```python
from build123d import *

# Parameters (mm, degrees)
F0_W     = 115
F0_H     = 65
F1_DEPTH = 5
F2_DEPTH = 5
F3_DEPTH = 10


with BuildPart() as f1:
    # F0 (on Top) → F1 (new body)
    with BuildSketch(Plane.XY):
        with Locations((-62.5, 32.5)):
            Rectangle(F0_W, F0_H)
    extrude(amount=F1_DEPTH)



with BuildPart() as f2:
    # F0 (on Top) → F2 (new body)
    with BuildSketch(Plane.XY):
        Polygon((-70, 70), (-50, 70), (-50, 100), (-60, 100), (-70, 100), align=None)
    extrude(amount=F2_DEPTH)


with BuildPart() as f2b:
    # F0 (on Top) → F2, piece 2 (new body)
    with BuildSketch(Plane.XY):
        Polygon((0, 45), (0, 25), (30, 25), (30, 35), (30, 45), align=None)
    extrude(amount=F2_DEPTH)


with BuildPart() as f1_1:
    add(f1.part)

    add(f2.part)  # F3 merges F2

    add(f2b.part)  # F3 merges F2b
    # F0 (on Top) → F3 (join)
    with BuildSketch(Plane.XY):
        Polygon((-5, 0), (0, 0), (0, 25), (0, 45), (0, 70), (-50, 70), (-70, 70), (-120, 70), (-120, 65), (-5, 65), align=None)
    extrude(amount=F3_DEPTH)


solid = f1_1.part
```
Could you check a few things on this model? Use its own coordinates, in mm. A direction names the side the tool comes from. Round coordinates to 2 decimals unless told otherwise and drop trailing zeros. Loops run counter-clockwise (first coordinate to the right, second up) from the corner with the lowest first, then second, coordinate; pieces in that order, holes last. Notation, with made-up numbers: (25.5, 48.25) - (77.5, 48.25) arc R24 ccw to (77.5, 59.25) - close; hole circle Ø4 at (46, 28.5). An arc over 180 degrees is marked (long way). Answer in a Markdown table with one row per item. Add a question column.
(1) For faces 1 (the face through (15, 25, 2)), 2 (the face through (-63, 65, 7)), 3 (the face through (15, 35, 5)), 4 (the face through (-60, 85, 5)), 5 (the face through (15, 45, 2)), which set-ups out of +Z, -Z, +X, -X, +Y, -Y let a thin tool reach every point of the face, with its end or its side?
(2) If we section it at A-A (z = 3.25): Please give me the cut outline in (x, y).
(3) If we section it at C-C (x = -98.5): Please give me the cut outline in (y, z).
(4) I need wall thicknesses on line 1 along Z through (x, y) = (-8, 37); line 2 along X through (y, z) = (36, 7.25); line 3 along Y through (x, z) = (-89, 1.25). Which ranges of each line are inside material? Lowest first, please.
(5) If we section it at B-B (y = 38): Please give me the cut outline in (x, z).
(6) If we section it at D-D (y = 21.5): Please give me the cut outline in (x, z).
(7) I'm going to push flat-ended pins straight in: pin 1 (2.5 mm diameter, centred on y = 89.5, z = 3.5, fed in from +X); pin 2 (6 mm diameter, centred on x = -9, z = 2.5, fed in from -Y); pin 3 (8 mm diameter, centred on x = -60.5, y = 28.5, fed in from +Z); pin 4 (2.5 mm diameter, centred on x = 19, z = 3.5, fed in from +Y). Where does each tip first touch, or does it pass through?
Model answer:
| question | item | result |
|---|---|---|
| 1 | face 1 | +Z, -Z, +X, -Y |
| 1 | face 2 | +Z, -X, -Y |
| 1 | face 3 | +Z, +X, +Y, -Y |
| 1 | face 4 | +Z, +X, -X, +Y |
| 1 | face 5 | +Z, -Z, +X, +Y |
| 2 | outline | (-120, 0) - (0, 0) - (0, 25) - (30, 25) - (30, 45) - (0, 45) - (0, 70) - (-50, 70) - (-50, 100) - (-70, 100) - (-70, 70) - (-120, 70) - close |
| 3 | outline | (0, 0) - (70, 0) - (70, 10) - (65, 10) - (65, 5) - (0, 5) - close |
| 4 | line 1 | z = 0 to 5 |
| 4 | line 2 | x = -5 to 0 |
| 4 | line 3 | y = 0 to 70 |
| 5 | outline | (-120, 0) - (30, 0) - (30, 5) - (0, 5) - (0, 10) - (-5, 10) - (-5, 5) - (-120, 5) - close |
| 6 | outline | (-120, 0) - (0, 0) - (0, 10) - (-5, 10) - (-5, 5) - (-120, 5) - close |
| 7 | pin 1 | stops at x = -50 |
| 7 | pin 2 | stops at y = 0 |
| 7 | pin 3 | stops at z = 5 |
| 7 | pin 4 | stops at y = 45 |
